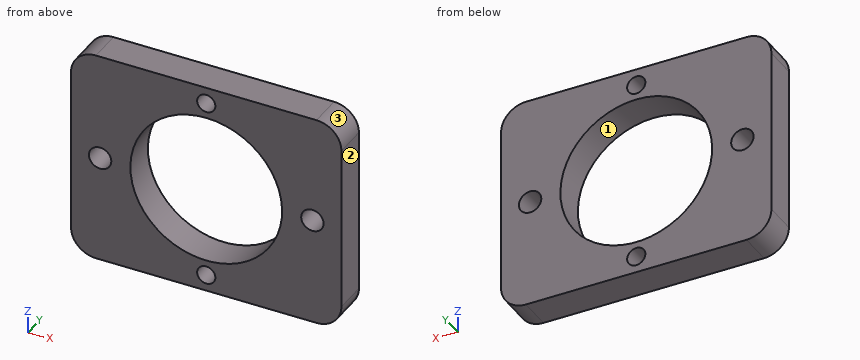
from build123d import *

# Parameters (mm, degrees)
SKETCH1_W           = 32.6
SKETCH1_H           = 26
BOSS_EXTRUDE1_DEPTH = 4
SKETCH2_R           = 9.15
SKETCH2_R_2         = 1.35
SKETCH2_R_3         = 1.1
CUT_EXTRUDE1_DEPTH  = 4
FILLET1_R           = 3


with BuildPart() as part:
    # Sketch1 → Boss-Extrude1 (new body)
    with BuildSketch(Plane(origin=(0, 0, 0), x_dir=(1, 0, 0), z_dir=(0, 1, 0))):
        with Locations((16.3, -13)):
            Rectangle(SKETCH1_W, SKETCH1_H)
    extrude(amount=BOSS_EXTRUDE1_DEPTH)

    # Sketch2 → Cut-Extrude1 (cut)
    with BuildSketch(Plane(origin=(0, 4, 0), x_dir=(1, 0, 0), z_dir=(0, 1, 0))):
        with Locations(Location((16.3, -13, 0), (0, 0, 270))):
            Circle(SKETCH2_R)
        with Locations(Location((3.5, -13, 0), (0, 0, 270))):
            Circle(SKETCH2_R_2)
        with Locations(Location((29.1, -13, 0), (0, 0, 270))):
            Circle(SKETCH2_R_2)
        with Locations(Location((16.3, -2, 0), (0, 0, 270))):
            Circle(SKETCH2_R_3)
        with Locations(Location((16.3, -24, 0), (0, 0, 270))):
            Circle(SKETCH2_R_3)
    extrude(amount=-CUT_EXTRUDE1_DEPTH, mode=Mode.SUBTRACT)

    # Fillet1
    fillet1_edges = [part.edges().sort_by_distance(p)[0] for p in [
        (0, 2, 0),
        (32.6, 2, 0),
        (32.6, 2, 26),
        (0, 2, 26),
    ]]
    fillet(fillet1_edges, radius=FILLET1_R)


solid = part.part
Can you work these out from the model? Positions are in its coordinate system, mm. Face numbers are marked on the shaded views. Round coordinates to 2 decimals unless told otherwise and drop trailing zeros. Write each loop counter-clockwise with the first axis right and the second up, starting at its lowest first coordinate (ties: lowest second). Pieces come first, ordered by that corner, then holes. Notation, with made-up numbers: M 65.25,39.25 L 77.25,39.25 A33 cw 77.25,67.25 Z; hole C 45.5,29 d5. An arc over 180 degrees is marked long. Use a Markdown table: item, result.
Item 1: We'd pull the mould along Z, two halves only. Please class the marked faces 1, 2 and 3: released by +Z, released by -Z, zero draft, split by the parting line, or undercut.
Found:
| item | result |
|---|---|
| face 1 | undercut |
| face 2 | zero draft |
| face 3 | released by +Z |
Item 2: I want a section at A-A (z = 13). List the corners of the cut face in (x, y) for me, and give its area (3 significant figures).
Found:
| item | result |
|---|---|
| outline | M 0,0 L 2.15,0 L 2.15,4 L 0,4 Z; M 4.85,0 L 7.15,0 L 7.15,4 L 4.85,4 Z; M 25.45,0 L 27.75,0 L 27.75,4 L 25.45,4 Z; M 30.45,0 L 32.6,0 L 32.6,4 L 30.45,4 Z |
| area | 35.6 mm2 |
Item 3: I want a section at C-C (x = 16.3). List the corners of the cut face in (y, z) for me.
Found:
| item | result |
|---|---|
| outline | M 0,0 L 4,0 L 4,0.9 L 0,0.9 Z; M 0,3.1 L 4,3.1 L 4,3.85 L 0,3.85 Z; M 0,22.15 L 4,22.15 L 4,22.9 L 0,22.9 Z; M 0,25.1 L 4,25.1 L 4,26 L 0,26 Z |
Item 4: For pin 1 Ø1.5 at (x, z) = (13.5, 20) entering from +Y; pin 2 Ø2.5 at (x, z) = (16.3, 24) entering from -Y, each with a flat end and sliding along its axis, tell me the tip position at first contact or that it passes through.
Found:
| item | result |
|---|---|
| pin 1 | passes through |
| pin 2 | stops at y = 0 |
Item 5: I want a section at D-D (x = 29.1). List the corners of the cut face in (y, z) for me.
Found:
| item | result |
|---|---|
| outline | M 0,0 L 4,0 L 4,11.65 L 0,11.65 Z; M 0,14.35 L 4,14.35 L 4,26 L 0,26 Z |
Item 6: I want a section at B-B (y = 2.15). List the corners of the cut face in (x, z) for me, and give its area (3 significant figures).
Found:
| item | result |
|---|---|
| outline | M 0,3 A3 ccw 3,0 L 29.6,0 A3 ccw 32.6,3 L 32.6,23 A3 ccw 29.6,26 L 3,26 A3 ccw 0,23 Z; hole C 3.5,13 d2.7; hole C 16.3,13 d18.3; hole C 16.3,2 d2.2; hole C 16.3,24 d2.2; hole C 29.1,13 d2.7 |
| area | 558 mm2 |
Item 7: If I drill on line 1 along X through (y, z) = (1.55, 13); line 2 along X through (y, z) = (0.75, 6); line 3 along X through (y, z) = (3.8, 8), over which ranges is the centre line in solid material (lowest first)? Write a range as [from, to].
Found:
| item | result |
|---|---|
| line 1 | x = [0, 2.15], [4.85, 7.15], [25.45, 27.75], [30.45, 32.6] |
| line 2 | x = [0, 10.41], [22.19, 32.6] |
| line 3 | x = [0, 8.64], [23.96, 32.6] |
